```python
from build123d import *

# Parameters (mm, degrees)
SKETCH_1_R          = 47.5
SKETCH_1_R_2        = 35
EXTRUDE_1_DEPTH     = 3
CUT_EXTRUDE_1_REACH = 69.242
SKETCH_2_R          = 2.15


with BuildPart() as part:
    # 草图1 → 凸台-拉伸1 (new body)
    with BuildSketch(Plane.XY):
        Circle(SKETCH_1_R)
        Circle(SKETCH_1_R_2, mode=Mode.SUBTRACT)
    extrude(amount=EXTRUDE_1_DEPTH)

    # 草图2 → 切除-拉伸1 (cut, up to next)
    with BuildSketch(Plane.XY.offset(3), mode=Mode.PRIVATE) as cut_extrude_1_sk1:
        with Locations((42.5, 0)):
            Circle(SKETCH_2_R)
    cut_extrude_1_tool1 = extrude(cut_extrude_1_sk1.sketch, amount=-CUT_EXTRUDE_1_REACH, mode=Mode.PRIVATE) & part.part
    # 草图2 → 切除-拉伸1 (cut, up to next)
    with BuildSketch(Plane.XY.offset(3), mode=Mode.PRIVATE) as cut_extrude_1_sk2:
        with Locations((0, -42.5)):
            Circle(SKETCH_2_R)
    cut_extrude_1_tool2 = extrude(cut_extrude_1_sk2.sketch, amount=-CUT_EXTRUDE_1_REACH, mode=Mode.PRIVATE) & part.part
    # 草图2 → 切除-拉伸1 (cut, up to next)
    with BuildSketch(Plane.XY.offset(3), mode=Mode.PRIVATE) as cut_extrude_1_sk3:
        with Locations((-42.5, 0)):
            Circle(SKETCH_2_R)
    cut_extrude_1_tool3 = extrude(cut_extrude_1_sk3.sketch, amount=-CUT_EXTRUDE_1_REACH, mode=Mode.PRIVATE) & part.part
    # 草图2 → 切除-拉伸1 (cut, up to next)
    with BuildSketch(Plane.XY.offset(3), mode=Mode.PRIVATE) as cut_extrude_1_sk4:
        with Locations((0, 42.5)):
            Circle(SKETCH_2_R)
    cut_extrude_1_tool4 = extrude(cut_extrude_1_sk4.sketch, amount=-CUT_EXTRUDE_1_REACH, mode=Mode.PRIVATE) & part.part
    add(cut_extrude_1_tool1.solids().sort_by_distance((42.5, 0, 3))[0], mode=Mode.SUBTRACT)
    add(cut_extrude_1_tool2.solids().sort_by_distance((0, -42.5, 3))[0], mode=Mode.SUBTRACT)
    add(cut_extrude_1_tool3.solids().sort_by_distance((-42.5, 0, 3))[0], mode=Mode.SUBTRACT)
    add(cut_extrude_1_tool4.solids().sort_by_distance((0, 42.5, 3))[0], mode=Mode.SUBTRACT)


solid = part.part
```
The model under review builds one solid part; all positions refer to its coordinate system, in mm. Give positions to 0.01 mm unless a question says otherwise; leave off trailing zeros. Loops run counter-clockwise (first coordinate to the right, second up) from the corner with the lowest first, then second, coordinate; pieces in that order, holes last. Notation, with made-up numbers: (51, -33.5) - (58, -33.5) arc R12 cw to (58, -22.5) - close; hole circle Ø11 at (-9, -20.5). An arc over 180 degrees is marked (long way). Answer as a JSON object with one key per item and string values.
Q1. Mouldability with a two-part tool opening along Y and no side actions: class faces 1 (the cylindrical face through (-0.28, -40.37, 1.52)), 2 (the cylindrical face through (-10.3, -46.37, 1.48)), 3 (the flat face through (3.3, 35.4, 0)) as +Y half, -Y half, draft (parallel to the pull), parting line (faces both ways), or undercut.
Worked out:
{"face 1": "undercut", "face 2": "parting line", "face 3": "draft"}
Q2. Add section C-C on x = 27. State the section outline as (y, z) points, plus the area to 3 significant figures.
Worked out:
{"outline": "(-39.08, 0) - (-22.27, 0) - (-22.27, 3) - (-39.08, 3) - close; (22.27, 0) - (39.08, 0) - (39.08, 3) - (22.27, 3) - close", "area": "101 mm^2"}
Q3. Add section A-A on x = 0. State the section outline as (y, z) points, plus the area to 3 significant figures.
Worked out:
{"outline": "(-47.5, 0) - (-44.65, 0) - (-44.65, 3) - (-47.5, 3) - close; (-40.35, 0) - (-35, 0) - (-35, 3) - (-40.35, 3) - close; (35, 0) - (40.35, 0) - (40.35, 3) - (35, 3) - close; (44.65, 0) - (47.5, 0) - (47.5, 3) - (44.65, 3) - close", "area": "49.2 mm^2"}
Q4. Insertion check: pin 1 (3.5 mm diameter, centred on x = 0, y = -42.5, fed in from -Z); pin 2 (1.5 mm diameter, centred on y = 6, z = 1, fed in from +X). Each pin has a flat end and moves straight along its axis. Give the tip position at first contact, or say it passes through.
Worked out:
{"pin 1": "passes through", "pin 2": "stops at x = 47.21"}
Q5. Add section B-B on y = 19.5. State the section outline as (x, z) points, plus the area to 3 significant figures.
Worked out:
{"outline": "(-43.31, 0) - (-29.06, 0) - (-29.06, 3) - (-43.31, 3) - close; (29.06, 0) - (43.31, 0) - (43.31, 3) - (29.06, 3) - close", "area": "85.5 mm^2"}
Q6. To check wall thickness, follow line 1 along Y through (x, z) = (0, 1.6); line 2 along Y through (x, z) = (42.5, 2.1); line 3 along Y through (x, z) = (28.5, 0.45). State the ranges of each line that lie inside material, in increasing order.
Worked out:
{"line 1": "y = -47.5 to -44.65, -40.35 to -35, 35 to 40.35, 44.65 to 47.5", "line 2": "y = -21.21 to -2.15, 2.15 to 21.21", "line 3": "y = -38 to -20.32, 20.32 to 38"}
